Check sheet for the modelled part. Datum: model origin and axes. Units: mm. A direction names the side the tool comes from. Round coordinates to 2 decimals unless told otherwise and drop trailing zeros. Order: outer loops, then holes, each group sorted by start corner. A loop starts at its lowest first (then second) coordinate and runs counter-clockwise, first axis right, second up. Notation, with made-up numbers: (-21.5, 68.25) -> (36.5, 68.25) arc R29 cw to (36.5, 94.25) -> close; hole circle Ø6 at (10.25, 80). An arc over 180 degrees is marked (long way). Answer in a Markdown table with one row per item.
Autodesk Inventor part; units mm, degrees
ref_plane "YZ Plane" through (0, 0, 0) normal (1, 0, 0) x (0, 1, 0)
ref_plane "XZ Plane" through (0, 0, 0) normal (0, 1, 0) x (-1, 0, 0)
ref_plane "XY Plane" through (0, 0, 0) normal (0, 0, 1) x (1, 0, 0)
sketch "Sketch1" plane through (0, 0, 0) normal (0, 0, 1) x (1, 0, 0)
  line L0 (0, 0) -> (620, 0)
  line L1 (620, 0) -> (620, 620)
  line L2 (620, 620) -> (0, 620)
  line L3 (0, 620) -> (0, 0)
  line L4 (203, 491) -> (417, 491)
  line L5 (417, 491) -> (417, 377)
  line L6 (417, 377) -> (203, 377)
  line L7 (203, 377) -> (203, 491)
  point P0 (310, 491)
  point P1 (310, 620)
  dimension "d0" = 620
  dimension "d1" = 620
  dimension "d2" = 214
  dimension "d3" = 114
  dimension "d4" = 129
extrude "Extrusion1" add sketch "Sketch1" along normal blind 10
sketch "Sketch2" plane through (0, 0, 10) normal (0, 0, 1) x (1, 0, 0)
  line L0 (0, 0) -> (310, 0)
  line L1 (310, 0) -> (310, 435)
  line L2 (310, 435) -> (0, 435)
  line L3 (0, 435) -> (0, 0)
  line L4 (620, 620) -> (0, 620)
  line L5 (0, 435) -> (620, 435)
  line L6 (620, 435) -> (620, 620)
  line L7 (620, 620) -> (0, 620)
  line L8 (0, 620) -> (0, 435)
  line L9 (310, 435) -> (620, 435)
  line L10 (620, 435) -> (620, 0)
  line L11 (620, 0) -> (310, 0)
  line L12 (310, 0) -> (310, 435)
  line L13 (620, 435) -> (310, 435)
  line L14 (310, 435) -> (310, 620)
  line L15 (310, 620) -> (620, 620)
  line L16 (620, 620) -> (620, 435)
  dimension "d7" = 435
extrude "Extrusion2" cut sketch "Sketch2" against normal through all contours L3 L2 L1 L0 | L1 L5 L10 L11 | L14 L4 L6 L5
sketch "Sketch6" plane through (0, 0, 10) normal (0, 0, 1) x (1, 0, 0)
  line L0 (310, 491) -> (310, 620)
  line L1 (310, 505.5) -> (295, 505.5)
  line L2 (295, 505.5) -> (295, 605.5)
  line L3 (295, 605.5) -> (310, 605.5)
  line L4 (310, 605.5) -> (310, 505.5)
  point P0 (0, 0)
  point P1 (310, 555.5)
  dimension "d30" = 15
  dimension "d31" = 100
extrude "Extrusion6" cut sketch "Sketch6" against normal blind 5
sketch "Sketch7" plane through (0, 0, 5) normal (0, 0, 1) x (1, 0, 0)
  line L0 (310, 605.5) -> (310, 505.5) construction
  line L1 (295, 605.5) -> (310, 605.5) construction
  line L2 (295, 505.5) -> (295, 605.5) construction
  line L3 (310, 505.5) -> (295, 505.5) construction
  circle A0 centre (302.5, 515.5) radius 2.5
  circle A1 centre (302.5, 595.5) radius 2.5
  point P0 (0, 0)
  point P1 (302.5, 605.5)
  point P2 (302.5, 505.5)
  dimension "d36" = 5
  dimension "d37" = 5
  dimension "d38" = 10
  dimension "d39" = 10
extrude "Extrusion7" cut sketch "Sketch7" against normal through all
sketch "Sketch8" plane through (0, 0, 10) normal (0, 0, 1) x (1, 0, 0)
  line L0 (203, 435) -> (0, 435)
  line L1 (27, 435) -> (176, 435)
  line L2 (176, 435) -> (176, 421)
  line L3 (176, 421) -> (27, 421)
  line L4 (27, 421) -> (27, 435)
  line L5 (26.5, 435) -> (176.5, 435) construction
  line L6 (176.5, 435) -> (176.5, 420) construction
  line L7 (176.5, 420) -> (26.5, 420) construction
  line L8 (26.5, 420) -> (26.5, 435) construction
  line L9 (0, 435) -> (203, 435)
  circle A0 centre (36.5, 427.5) radius 2.5
  circle A1 centre (166.5, 427.5) radius 2.5
  point P0 (0, 0)
  point P1 (101.5, 435)
  point P2 (101.5, 435)
  point P3 (176.5, 427.5)
  point P4 (26.5, 427.5)
  dimension "d44" = 149
  dimension "d45" = 14
  dimension "d46" = 150
  dimension "d47" = 15
  dimension "d48" = 5
  dimension "d49" = 5
  dimension "d50" = 10
  dimension "d51" = 10
extrude "Extrusion8" add sketch "Sketch8" against normal blind 5
properties part number "TC001b" material "ABS Plastic"
Item 1: Cross-section at B-B (y = 479.5). Record the boundary of the cut face in (x, z).
Result sheet:
| item | result |
|---|---|
| outline | (0, 0) -> (203, 0) -> (203, 10) -> (0, 10) -> close |
Item 2: Scan lines: line 1 (X direction, y = 427.5, z = 6.65); line 2 (Y direction, x = 302.5, z = 1.8); line 3 (Y direction, x = 166.5, z = 8.5). Record each from-to range of solid material in increasing order. Write a range as [from, to].
Result sheet:
| item | result |
|---|---|
| line 1 | x = [27, 34], [39, 164], [169, 176] |
| line 2 | y = [491, 513], [518, 593], [598, 620] |
| line 3 | y = [421, 425], [430, 620] |
Item 3: Cross-section at A-A (z = 8). Record the boundary of the cut face in (x, y).
Result sheet:
| item | result |
|---|---|
| outline | (0, 435) -> (27, 435) -> (27, 421) -> (176, 421) -> (176, 435) -> (203, 435) -> (203, 491) -> (310, 491) -> (310, 505.5) -> (295, 505.5) -> (295, 605.5) -> (310, 605.5) -> (310, 620) -> (0, 620) -> close; hole circle Ø5 at (36.5, 427.5); hole circle Ø5 at (166.5, 427.5) |
Item 4: Set-up check for faces 1 (the flat face through (100, 428, 5)), 2 (the flat face through (153, 529, 0)), 3 (the flat face through (302, 556, 5)), 4 (the flat face through (256, 491, 5)), 5 (the flat face through (310, 555, 3)): record each of +Z, -Z, +X, -X, +Y, -Y from which the full face is reachable in a straight line by a thin tool's end or side.
Result sheet:
| item | result |
|---|---|
| face 1 | -Z, +X, -X, -Y |
| face 2 | -Z, +X, -X, +Y, -Y |
| face 3 | +Z, +X |
| face 4 | +Z, -Z, +X, -Y |
| face 5 | +Z, -Z, +X, +Y, -Y |
Item 5: Depth check by flat-ended pin: P1, Ø3, axis at x = 302.5, y = 515.5, coming from the +Z side; P2, Ø4, axis at y = 542.5, z = 8.5, coming from the +X side; P3, Ø4, axis at y = 429.5, z = 7, coming from the +X side; P4, Ø16.5, axis at x = 305.5, y = 561, coming from the +Z side. Enter the tip coordinate at first touch or a pass-through.
Result sheet:
| item | result |
|---|---|
| P1 | passes through |
| P2 | stops at x = 295 |
| P3 | stops at x = 176 |
| P4 | stops at z = 5 |
Item 6: Cross-section at D-D (y = 571). Record the boundary of the cut face in (x, z), and give its area (4 significant figures).
Result sheet:
| item | result |
|---|---|
| outline | (0, 0) -> (310, 0) -> (310, 5) -> (295, 5) -> (295, 10) -> (0, 10) -> close |
| area | 3,025 mm^2 |
Item 7: Cross-section at C-C (x = 233). Record the boundary of the cut face in (y, z).
Result sheet:
| item | result |
|---|---|
| outline | (491, 0) -> (620, 0) -> (620, 10) -> (491, 10) -> close |
